The model under review builds one solid part; all positions refer to its coordinate system, in mm. A direction names the side the tool comes from. Give positions to 0.01 mm unless a question says otherwise; leave off trailing zeros. Loops run counter-clockwise (first coordinate to the right, second up) from the corner with the lowest first, then second, coordinate; pieces in that order, holes last. Notation, with made-up numbers: M 38.25,64.5 L 44.25,64.5 A26 ccw 44.25,86.5 Z; hole C 14.25,-22 d8. An arc over 180 degrees is marked long. Return JSON: item names as keys, results as strings.
```python
from build123d import *

# Parameters (mm, degrees)
SKETCH1_W                                         = 73.66
SKETCH1_H                                         = 69.85
BOSS_EXTRUDE1_DEPTH                               = 8.89
SKETCH2_R                                         = 2.032
CUT_EXTRUDE1_DEPTH                                = 8.89
SKETCH3_W                                         = 73.66
SKETCH3_H                                         = 12.7
BOSS_EXTRUDE2_DEPTH                               = 127
BOSS_EXTRUDE3_DEPTH                               = 38.1
BOSS_EXTRUDE3_DEPTH_BACK                          = 135.89
SKETCH4_W                                         = 73.66
SKETCH4_H                                         = 12.7
BOSS_EXTRUDE4_START                               = -36.83
BOSS_EXTRUDE4_DEPTH                               = 6.35
SKETCH7_R                                         = 2.667
SKETCH7_R_2                                       = 5.207
SKETCH7_R_3                                       = 2.413
CUT_EXTRUDE2_DEPTH                                = 12.7
SKETCH27_W                                        = 12.3952
SKETCH27_H                                        = 6.35
CUT_EXTRUDE3_DEPTH                                = 12.7
SKETCH28_W                                        = 12.3952
SKETCH28_H                                        = 6.35
CUT_EXTRUDE4_DEPTH                                = 12.7
CSK_FOR_6_FLAT_HEAD_MACHINE_SCREW_100_D           = 3.7973
CSK_FOR_6_FLAT_HEAD_MACHINE_SCREW_100_CSINK_D     = 7.0866
CSK_FOR_6_FLAT_HEAD_MACHINE_SCREW_100_CSINK_ANGLE = 100
FILLET1_R                                         = 5.08
SKETCH35_R                                        = 5.08
CUT_EXTRUDE5_DEPTH                                = 6.35


with BuildPart() as part:
    # Sketch1 → Boss-Extrude1 (new body)
    with BuildSketch(Plane.XY):
        Rectangle(SKETCH1_W, SKETCH1_H)
    extrude(amount=BOSS_EXTRUDE1_DEPTH)

    # Sketch2 → Cut-Extrude1 (cut)
    with BuildSketch(Plane(origin=(0, 0, 0), x_dir=(-1, 0, 0), z_dir=(0, 0, -1))):
        with Locations((-29.9085, 29.845)):
            Circle(SKETCH2_R)
        with Locations((-29.9085, 12.065)):
            Circle(SKETCH2_R)
        with Locations(Location((29.9085, 12.065, 0), (0, 0, 180))):
            Circle(SKETCH2_R)
        with Locations(Location((29.9085, 29.845, 0), (0, 0, 180))):
            Circle(SKETCH2_R)
    extrude(amount=-CUT_EXTRUDE1_DEPTH, mode=Mode.SUBTRACT)

    # Sketch3 → Boss-Extrude2 (add)
    with BuildSketch(Plane(origin=(0, 0, 0), x_dir=(-1, 0, 0), z_dir=(0, 0, -1))):
        with Locations((0, -34.925)):
            Rectangle(SKETCH3_W, SKETCH3_H)
    extrude(amount=BOSS_EXTRUDE2_DEPTH)

    # Sketch4 → Boss-Extrude3 (add, two sides: drawn at the far end of the back side and taken through both)
    with BuildSketch(Plane.XY.offset(8.89).offset(-BOSS_EXTRUDE3_DEPTH_BACK)):
        with Locations((0, -34.925)):
            Rectangle(SKETCH4_W, SKETCH4_H)
    extrude(amount=BOSS_EXTRUDE3_DEPTH + BOSS_EXTRUDE3_DEPTH_BACK)

    # Sketch5 → Boss-Extrude4 (add, symmetric)
    with BuildSketch(Plane(origin=(36.83, 0, 0), x_dir=(0, 0, -1), z_dir=(1, 0, 0)).offset(BOSS_EXTRUDE4_START)):
        Polygon((-46.99, -28.575), (-8.89, 25.837439057), (-8.89, -28.575), align=None)
    extrude(amount=BOSS_EXTRUDE4_DEPTH, both=True)

    # Sketch7 → Cut-Extrude2 (cut)
    with BuildSketch(Plane(origin=(0, -28.575, 0), x_dir=(1, 0, 0), z_dir=(0, 1, 0))):
        with Locations(Location((0, 26.416, 0), (0, 0, 270))):
            Circle(SKETCH7_R)
        with Locations(Location((0, 89.916, 0), (0, 0, 270))):
            Circle(SKETCH7_R_2)
        with Locations(Location((-20.32, 69.596, 0), (0, 0, 270))):
            Circle(SKETCH7_R_3)
        with Locations(Location((20.32, 69.596, 0), (0, 0, 270))):
            Circle(SKETCH7_R_3)
        with Locations(Location((20.32, 110.236, 0), (0, 0, 270))):
            Circle(SKETCH7_R_3)
        with Locations(Location((-20.32, 110.236, 0), (0, 0, 270))):
            Circle(SKETCH7_R_3)
    extrude(amount=-CUT_EXTRUDE2_DEPTH, mode=Mode.SUBTRACT)

    # Sketch27 → Cut-Extrude3 (cut)
    with BuildSketch(Plane.ZY.offset(36.83)):
        with Locations((-19.2024, -31.75)):
            Rectangle(SKETCH27_W, SKETCH27_H)
    extrude(amount=-CUT_EXTRUDE3_DEPTH, mode=Mode.SUBTRACT)

    # Sketch28 → Cut-Extrude4 (cut)
    with BuildSketch(Plane(origin=(36.83, 0, 0), x_dir=(0, 0, -1), z_dir=(1, 0, 0))):
        with Locations((19.2024, -31.75)):
            Rectangle(SKETCH28_W, SKETCH28_H)
    extrude(amount=-CUT_EXTRUDE4_DEPTH, mode=Mode.SUBTRACT)

    # CSK for #6 Flat Head Machine Screw (100)1 (through all)
    with Locations(Plane(origin=(0, -28.575, 0), x_dir=(1, 0, 0), z_dir=(0, 1, 0))):
        with Locations((-29.21, -39.37), (29.21, -39.37), (29.21, 119.38), (-29.21, 119.38)):
            CounterSinkHole(CSK_FOR_6_FLAT_HEAD_MACHINE_SCREW_100_D / 2, CSK_FOR_6_FLAT_HEAD_MACHINE_SCREW_100_CSINK_D / 2, counter_sink_angle=CSK_FOR_6_FLAT_HEAD_MACHINE_SCREW_100_CSINK_ANGLE)

    # Fillet1
    fillet1_edges = [part.edges().sort_by_distance(p)[0] for p in [
        (0, -28.575, 0),
    ]]
    fillet(fillet1_edges, radius=FILLET1_R)
    fillet1_2_edges = [part.edges().sort_by_distance(p)[0] for p in [
        (-6.35, -1.368780472, 8.89),
    ]]
    fillet(fillet1_2_edges, radius=FILLET1_R)
    fillet1_3_edges = [part.edges().sort_by_distance(p)[0] for p in [
        (6.35, -1.368780472, 8.89),
    ]]
    fillet(fillet1_3_edges, radius=FILLET1_R)
    fillet1_4_edges = [part.edges().sort_by_distance(p)[0] for p in [
        (0, 25.837439057, 8.89),
    ]]
    fillet(fillet1_4_edges, radius=FILLET1_R)
    fillet1_5_edges = [part.edges().sort_by_distance(p)[0] for p in [
        (36.83, -34.925, -127),
    ]]
    fillet(fillet1_5_edges, radius=FILLET1_R)
    fillet1_6_edges = [part.edges().sort_by_distance(p)[0] for p in [
        (36.83, -34.925, 46.99),
    ]]
    fillet(fillet1_6_edges, radius=FILLET1_R)
    fillet1_7_edges = [part.edges().sort_by_distance(p)[0] for p in [
        (-36.83, -34.925, 46.99),
    ]]
    fillet(fillet1_7_edges, radius=FILLET1_R)
    fillet1_8_edges = [part.edges().sort_by_distance(p)[0] for p in [
        (-36.83, -34.925, -127),
    ]]
    fillet(fillet1_8_edges, radius=FILLET1_R)
    # the kernel refuses this fillet: 5.08 mm, written as the material it adds along each edge
    with BuildSketch(Plane(origin=(6.35, -28.575, 13.97), x_dir=(1, 0, 0), z_dir=(0, 0, 1))) as fillet1_9_piece_1_section:
        with BuildLine():
            CenterArc((FILLET1_R, FILLET1_R), FILLET1_R, 180, 90)
            Line((0, FILLET1_R), (-FILLET1_R * 0.02, FILLET1_R))
            Line((-FILLET1_R * 0.02, FILLET1_R), (-FILLET1_R * 0.02, -FILLET1_R * 0.02))
            Line((-FILLET1_R * 0.02, -FILLET1_R * 0.02), (FILLET1_R, -FILLET1_R * 0.02))
            Line((FILLET1_R, -FILLET1_R * 0.02), (FILLET1_R, 0))
        make_face()
    fillet1_9_piece_1 = extrude(amount=33.02, mode=Mode.PRIVATE)
    fillet1_9_piece_1 = split(fillet1_9_piece_1, bisect_by=Plane(origin=(7.515371232, -19.877941852, 40.900254324), z_dir=(0, -0.5735764363510472, -0.8191520442889911)), keep=Keep.TOP, mode=Mode.PRIVATE)
    add(fillet1_9_piece_1)
    with BuildSketch(Plane(origin=(11.43, -28.575, 13.97), x_dir=(0, 0, -1), z_dir=(1, 0, 0))) as fillet1_9_piece_2:
        with BuildLine():
            CenterArc((5.08 - FILLET1_R, FILLET1_R), FILLET1_R, 270, 90)
            Line((5.08, FILLET1_R), (5.08 + FILLET1_R * 0.02, FILLET1_R))
            Line((5.08 + FILLET1_R * 0.02, FILLET1_R), (5.08 + FILLET1_R * 0.02, 0))
            Line((5.08 + FILLET1_R * 0.02, 0), (5.08, -FILLET1_R * 0.02))
            Line((5.08, -FILLET1_R * 0.02), (5.08 - FILLET1_R, -FILLET1_R * 0.02))
            Line((5.08 - FILLET1_R, -FILLET1_R * 0.02), (5.08 - FILLET1_R, 0))
        make_face()
    revolve(axis=Axis((11.43, -28.575, 13.97), (0, 1, 0)), revolution_arc=90)
    with BuildSketch(Plane(origin=(11.43, -28.575, 8.89), x_dir=(0, 1, 0), z_dir=(1, 0, 0))) as fillet1_9_piece_3:
        with BuildLine():
            CenterArc((FILLET1_R, FILLET1_R), FILLET1_R, 180, 90)
            Line((0, FILLET1_R), (-FILLET1_R * 0.02, FILLET1_R))
            Line((-FILLET1_R * 0.02, FILLET1_R), (-FILLET1_R * 0.02, -FILLET1_R * 0.02))
            Line((-FILLET1_R * 0.02, -FILLET1_R * 0.02), (FILLET1_R, -FILLET1_R * 0.02))
            Line((FILLET1_R, -FILLET1_R * 0.02), (FILLET1_R, 0))
        make_face()
    extrude(amount=25.4)
    # the kernel refuses this fillet: 5.08 mm, written as the material it adds along each edge
    with BuildSketch(Plane(origin=(-6.35, -28.575, 13.97), x_dir=(-1, 0, 0), z_dir=(0, 0, 1))) as fillet1_10_piece_1_section:
        with BuildLine():
            CenterArc((FILLET1_R, -FILLET1_R), FILLET1_R, 90, 90)
            Line((0, -FILLET1_R), (-FILLET1_R * 0.02, -FILLET1_R))
            Line((-FILLET1_R * 0.02, -FILLET1_R), (-FILLET1_R * 0.02, FILLET1_R * 0.02))
            Line((-FILLET1_R * 0.02, FILLET1_R * 0.02), (FILLET1_R, FILLET1_R * 0.02))
            Line((FILLET1_R, FILLET1_R * 0.02), (FILLET1_R, 0))
        make_face()
    fillet1_10_piece_1 = extrude(amount=33.02, mode=Mode.PRIVATE)
    fillet1_10_piece_1 = split(fillet1_10_piece_1, bisect_by=Plane(origin=(-7.515371232, -19.877941852, 40.900254324), z_dir=(0, -0.5735764363510472, -0.8191520442889911)), keep=Keep.TOP, mode=Mode.PRIVATE)
    add(fillet1_10_piece_1)
    with BuildSketch(Plane(origin=(-11.43, -28.575, 13.97), x_dir=(0, 0, -1), z_dir=(-1, 0, 0))) as fillet1_10_piece_2:
        with BuildLine():
            CenterArc((5.08 - FILLET1_R, -FILLET1_R), FILLET1_R, 0, 90)
            Line((5.08, -FILLET1_R), (5.08 + FILLET1_R * 0.02, -FILLET1_R))
            Line((5.08 + FILLET1_R * 0.02, -FILLET1_R), (5.08 + FILLET1_R * 0.02, 0))
            Line((5.08 + FILLET1_R * 0.02, 0), (5.08, FILLET1_R * 0.02))
            Line((5.08, FILLET1_R * 0.02), (5.08 - FILLET1_R, FILLET1_R * 0.02))
            Line((5.08 - FILLET1_R, FILLET1_R * 0.02), (5.08 - FILLET1_R, 0))
        make_face()
    revolve(axis=Axis((-11.43, -28.575, 13.97), (0, -1, 0)), revolution_arc=90)
    with BuildSketch(Plane(origin=(-36.83, -28.575, 8.89), x_dir=(0, 0, 1), z_dir=(1, 0, 0))) as fillet1_10_piece_3:
        with BuildLine():
            CenterArc((FILLET1_R, -FILLET1_R), FILLET1_R, 90, 90)
            Line((0, -FILLET1_R), (-FILLET1_R * 0.02, -FILLET1_R))
            Line((-FILLET1_R * 0.02, -FILLET1_R), (-FILLET1_R * 0.02, FILLET1_R * 0.02))
            Line((-FILLET1_R * 0.02, FILLET1_R * 0.02), (FILLET1_R, FILLET1_R * 0.02))
            Line((FILLET1_R, FILLET1_R * 0.02), (FILLET1_R, 0))
        make_face()
    extrude(amount=25.4)

    # Sketch35 → Cut-Extrude5 (cut)
    with BuildSketch(Plane.XZ.offset(41.275)):
        with Locations((20.32, -110.236)):
            Circle(SKETCH35_R)
        with Locations((-20.32, -110.236)):
            Circle(SKETCH35_R)
        with Locations((-20.32, -69.596)):
            Circle(SKETCH35_R)
        with Locations((20.32, -69.596)):
            Circle(SKETCH35_R)
    extrude(amount=-CUT_EXTRUDE5_DEPTH, mode=Mode.SUBTRACT)


solid = part.part
```
1) Wall thickness on L1, parallel to Z at x = 29, y = -35; L2, parallel to Z at x = 29, y = -34; L3, parallel to Z at x = -20.32, y = -37: over which ranges is each line inside the solid? List them lowest first. Write a range as from..to.
From the geometry:
{"L1": "-127..-121.27, -117.49..37.48, 41.26..46.99", "L2": "-127..-121.27, -117.49..-25.4, -13..37.48, 41.26..46.99", "L3": "-127..-115.32, -105.16..-74.68, -64.52..46.99"}
2) Consider section C-C on z = -89. Write out the cut boundary in (x, y) (3 decimals).
From the geometry:
{"outline": "M -36.83,-41.275 L -5.126,-41.275 L -5.126,-28.575 L -36.83,-28.575 Z; M 5.126,-41.275 L 36.83,-41.275 L 36.83,-28.575 L 5.126,-28.575 Z"}
3) Insertion check: pin 1 (13.5 mm diameter, centred on x = 29.5, z = -20.5, fed in from +Y) (3 decimals); pin 2 (3.5 mm diameter, centred on x = 29.91, y = 29.84, fed in from -Z); pin 3 (6 mm diameter, centred on x = -20.32, z = -69.596, fed in from -Y) (3 decimals); pin 4 (4 mm diameter, centred on x = 19.5, y = -20.5, fed in from -Z). Each pin has a flat end and moves straight along its axis. Give the tip position at first contact, or say it passes through.
From the geometry:
{"pin 1": "y = -28.575", "pin 2": "through", "pin 3": "y = -34.925", "pin 4": "z = 0"}
4) Consider section D-D on y = -0.5. Write out the cut boundary in (x, z), then the cut area to 3 significant figures.
From the geometry:
{"outline": "M -36.83,0 L 36.83,0 L 36.83,8.89 L 11.43,8.89 A5.08 cw 6.35,13.97 L 6.35,27.33 L -6.35,27.33 L -6.35,13.97 A5.08 cw -11.43,8.89 L -36.83,8.89 Z", "area": "900 mm²"}
5) The part is to be moulded in two halves that separate along X. For faces 1 (the face through (-18, -34.925, -71)), 2 (the face through (35.381, -34.836, 45.462)), 3 (the face through (-35.381, -34.836, -125.472)), 4 (the face through (0, -35, -127)), say which applies: released by +X, released by -X, zero draft, split by the parting line, or undercut.
From the geometry:
{"face 1": "undercut", "face 2": "released by +X", "face 3": "released by -X", "face 4": "zero draft"}
6) Consider section B-B on x = 20.32. Write out the cut boundary in (y, z) (3 decimals), then the cut area to 3 significant figures.
From the geometry:
{"outline": "M -41.275,-127 L -28.575,-127 L -28.575,-112.649 L -34.925,-112.649 L -34.925,-115.316 L -41.275,-115.316 Z; M -41.275,-105.156 L -34.925,-105.156 L -34.925,-107.823 L -28.575,-107.823 L -28.575,-72.009 L -34.925,-72.009 L -34.925,-74.676 L -41.275,-74.676 Z; M -41.275,-64.516 L -34.925,-64.516 L -34.925,-67.183 L -28.575,-67.183 L -28.575,-5.08 A5.08 cw -23.495,0 L 34.925,0 L 34.925,8.89 L -23.495,8.89 A5.08 cw -28.575,13.97 L -28.575,46.99 L -41.275,46.99 Z", "area": "2,590 mm²"}
7) Tool access review of faces 5 (the face through (-24.31, -27.13, 10.42)), 6 (the face through (-31, -32, -25.4)), 7 (the face through (31, -32, -13.005)), 8 (the face through (6.35, -12, 22)), 9 (the face through (-1, 6, 0)): name each direction out of +Z, -Z, +X, -X, +Y, -Y from which nothing blocks a thin tool from reaching the whole face with its end or side.
From the geometry:
{"face 5": "+Z, -X, +Y", "face 6": "-X, +Y", "face 7": "+X, +Y", "face 8": "+Z, +X, +Y", "face 9": "-Z, +X, -X, +Y"}
8) Consider section A-A on z = -119.38. Write out the cut boundary in (x, y) (3 decimals).
From the geometry:
{"outline": "M -36.83,-41.275 L -31.109,-41.275 L -31.109,-29.955 L -32.753,-28.575 L -36.83,-28.575 Z; M -27.311,-41.275 L 27.311,-41.275 L 27.311,-29.955 L 25.667,-28.575 L -25.667,-28.575 L -27.311,-29.955 Z; M 31.109,-41.275 L 36.83,-41.275 L 36.83,-28.575 L 32.753,-28.575 L 31.109,-29.955 Z"}
